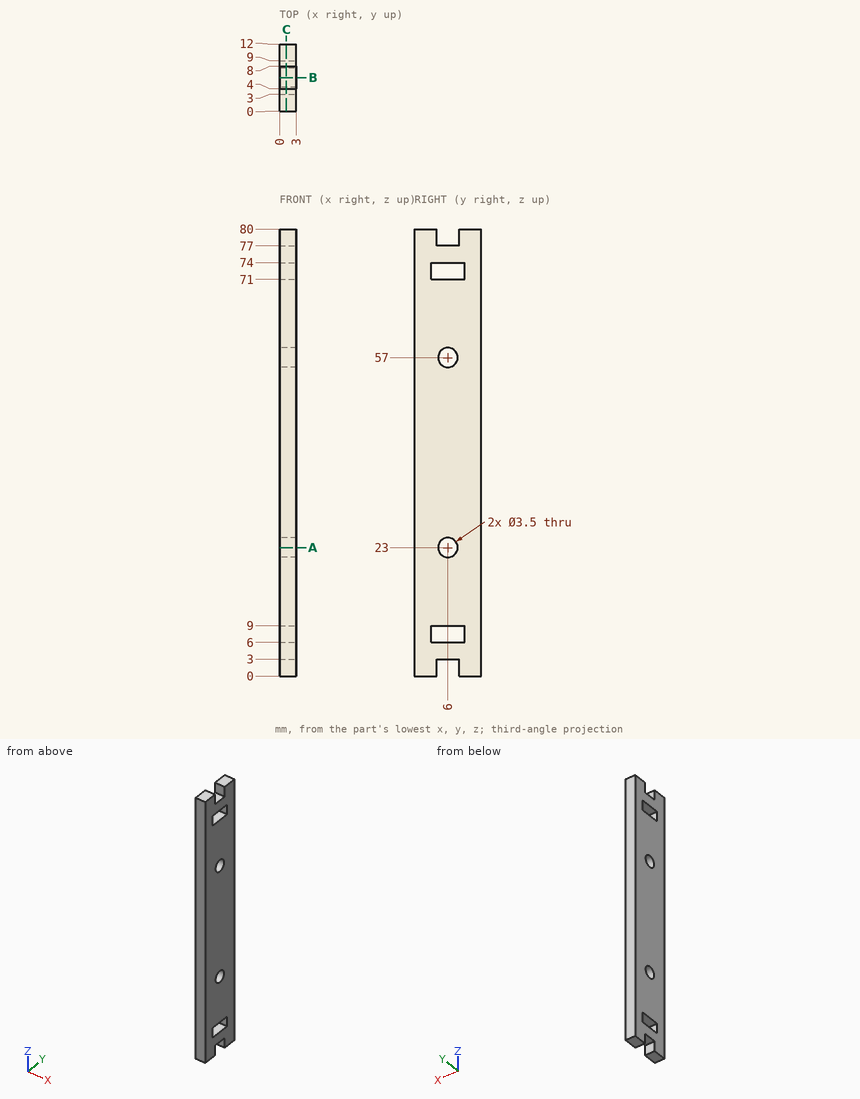
Can you work these out from the drawing? Everything is in mm from the part's minimum corner. Give positions to 0.01 mm unless a question says otherwise; leave off trailing zeros. Loops run counter-clockwise (first coordinate to the right, second up) from the corner with the lowest first, then second, coordinate; pieces in that order, holes last. Notation, with made-up numbers: (23, 53) -> (38, 53) arc R17 cw to (38, 57) -> close; hole circle Ø11 at (14, 80.25). An arc over 180 degrees is marked (long way). Return JSON: item names as keys, results as strings.
Q1. I want a section at C-C, the plane x = 1.2. List the corners of the cut face in (y, z) for me, then the cut area to 3 significant figures.
Checks:
{"outline": "(0, 0) -> (4, 0) -> (4, 3) -> (8, 3) -> (8, 0) -> (12, 0) -> (12, 80) -> (8, 80) -> (8, 77) -> (4, 77) -> (4, 80) -> (0, 80) -> close; hole (3, 6) -> (9, 6) -> (9, 9) -> (3, 9) -> close; hole (3, 71) -> (9, 71) -> (9, 74) -> (3, 74) -> close; hole circle Ø3.5 at (6, 23); hole circle Ø3.5 at (6, 57)", "area": "881 mm2"}
Q2. I want a section at B-B, the plane y = 6. List the corners of the cut face in (x, z) for me.
Checks:
{"outline": "(0, 3) -> (3, 3) -> (3, 6) -> (0, 6) -> close; (0, 9) -> (3, 9) -> (3, 21.25) -> (0, 21.25) -> close; (0, 24.75) -> (3, 24.75) -> (3, 55.25) -> (0, 55.25) -> close; (0, 58.75) -> (3, 58.75) -> (3, 71) -> (0, 71) -> close; (0, 74) -> (3, 74) -> (3, 77) -> (0, 77) -> close"}
Q3. For pin 1 Ø3 at (y, z) = (6, 57) entering from +X; pin 2 Ø1.5 at (x, y) = (1.5, 6) entering from +Z; pin 3 Ø1.5 at (x, y) = (2, 5.5) entering from -Z, each with a flat end and sliding along its axis, tell me the tip position at first contact or that it passes through.
Checks:
{"pin 1": "passes through", "pin 2": "stops at z = 77", "pin 3": "stops at z = 3"}
Q4. I want a section at A-A, the plane z = 23. List the corners of the cut face in (x, y) for me, then the cut area to 3 significant figures.
Checks:
{"outline": "(0, 0) -> (3, 0) -> (3, 4.25) -> (0, 4.25) -> close; (0, 7.75) -> (3, 7.75) -> (3, 12) -> (0, 12) -> close", "area": "25.5 mm2"}
Q5. I need wall thicknesses on probe 1 along Z at (x, y) = (0.9, 6); probe 2 along Z at (x, y) = (1.7, 8.75); probe 3 along Y at (x, z) = (2.85, 73.5). Which ranges of each line are inside material? Lowest first, please.
Checks:
{"probe 1": "z = 3 to 6, 9 to 21.25, 24.75 to 55.25, 58.75 to 71, 74 to 77", "probe 2": "z = 0 to 6, 9 to 71, 74 to 80", "probe 3": "y = 0 to 3, 9 to 12"}
